For this review, take the finished solid that the model builds, in its own axes (mm). A direction names the side the tool comes from. Round coordinates to 2 decimals unless told otherwise and drop trailing zeros. Write each loop counter-clockwise with the first axis right and the second up, starting at its lowest first coordinate (ties: lowest second). Pieces come first, ordered by that corner, then holes. Notation, with made-up numbers: M 7.5,-2 L 14.5,-2 A3 ccw 14.5,2 Z; hole C 70.25,7 d11. An arc over 180 degrees is marked long. Answer in a Markdown table with one row per item.
Autodesk Inventor part; units mm, degrees
ref_plane "YZ Plane" through (0, 0, 0) normal (1, 0, 0) x (0, 1, 0)
ref_plane "XZ Plane" through (0, 0, 0) normal (0, 1, 0) x (-1, 0, 0)
ref_plane "XY Plane" through (0, 0, 0) normal (0, 0, 1) x (1, 0, 0)
sketch "Sketch2" plane through (0, 0, 0) normal (0, 1, 0) x (-1, 0, 0)
  circle A0 centre (0, 0) radius 10
  dimension "d0" = 20
extrude "Extrusion1" add sketch "Sketch2" along normal blind 20
sketch "Sketch3" plane through (0, 0, 0) normal (0, -1, 0) x (1, 0, 0)
  circle A0 centre (0, 0) radius 4.15
  dimension "d3" = 8.3
extrude "Extrusion2" cut sketch "Sketch3" against normal blind 12.4
sketch "Sketch4" plane through (0, 12.4, 0) normal (0, -1, 0) x (1, 0, 0)
  circle A0 centre (0, 0) radius 4.15
  circle A1 centre (0, 0) radius 3.2
  line L0 (3.2, 0) -> (-1.7, 0)
  line L1 (-1.7, 0) -> (-1.7, -3.7858)
  line L2 (-1.7, 0) -> (-1.7, 3.7858)
  point P0 (-1.7, 2.7111)
  point P1 (-1.7, -2.7111)
  dimension "d16" = 6.4
  dimension "d17" = 4.9
extrude "Extrusion3" cut sketch "Sketch4" against normal blind 6.7 contours A1 L0 L2 | L1 L0 A1
sketch "Sketch8" plane through (0, 0, 0) normal (0, -1, 0) x (1, 0, 0)
  circle A0 centre (0, 0) radius 9.1
  dimension "d18" = 18.2
extrude "Extrusion7" cut sketch "Sketch8" against normal blind 4.5
sketch "Sketch9" plane through (0, 0, 0) normal (0, -1, 0) x (1, 0, 0)
  circle A0 centre (0, 0) radius 10
extrude "Extrusion8" cut sketch "Sketch9" against normal blind 2.8
sketch "Sketch10" plane through (0, 12.4, 0) normal (0, -1, 0) x (1, 0, 0)
  arc A0 (-1.7, -2.7111) -> (-1.7, 2.7111) centre (0, 0) ccw
  line L0 (-1.7, -2.7111) -> (-1.7, 2.7111)
  circle A1 centre (0, 0) radius 4.15
extrude "Extrusion9" cut sketch "Sketch10" against normal blind 0.4
properties part number "RotaryEncoderKnob"
Q1. Take a section at D-D (z = -7.75). State the section outline as (x, y) points, then the cut area to 3 significant figures.
Found:
| item | result |
|---|---|
| outline | M -6.32,2.8 L -4.77,2.8 L -4.77,4.5 L 4.77,4.5 L 4.77,2.8 L 6.32,2.8 L 6.32,20 L -6.32,20 Z |
| area | 201 mm² |
Q2. Take a section at A-A (y = 6.5). State the section outline as (x, z) points.
Found:
| item | result |
|---|---|
| outline | C 0,0 d20; hole C 0,0 d8.3 |
Q3. Take a section at B-B (z = 0). State the section outline as (x, y) points, then the cut area to 3 significant figures.
Found:
| item | result |
|---|---|
| outline | M -10,2.8 L -9.1,2.8 L -9.1,4.5 L -4.15,4.5 L -4.15,12.8 L -1.7,12.8 L -1.7,19.1 L 3.2,19.1 L 3.2,12.8 L 4.15,12.8 L 4.15,4.5 L 9.1,4.5 L 9.1,2.8 L 10,2.8 L 10,20 L -10,20 Z |
| area | 213 mm² |
Q4. Mouldability with a two-part tool opening along X and no side actions: class faces 3 (the face through (2.17, 11.28, 9.76)), 4 (the face through (-4.5, 2.8, -8.1)), 5 (the face through (-1.973, 3.638, -8.884)) as +X half, -X half, draft (parallel to the pull), parting line (faces both ways), or undercut.
Found:
| item | result |
|---|---|
| face 3 | parting line |
| face 4 | draft |
| face 5 | undercut |
Q5. For probe 1 along Z at (x, y) = (0, 8.75); probe 2 along X at (y, z) = (10.75, 0.25); probe 3 along Z at (x, y) = (0, 3.35), list the stretches that pass through material, from the lowest coordinate up.
Found:
| item | result |
|---|---|
| probe 1 | -10 to -4.15, 4.15 to 10 |
| probe 2 | -10 to -4.14, 4.14 to 10 |
| probe 3 | -10 to -9.1, 9.1 to 10 |
Q6. Machinability: for faces 1 (the face through (0, 20, 0)), 2 (the face through (2, 4.5, -4)), which of the approach directions +Z, -Z, +X, -X, +Y, -Y give a long, thin tool a straight path to every point of the face, cutting with its end or side? Answer none if there is none.
Found:
| item | result |
|---|---|
| face 1 | +Z, -Z, +X, -X, +Y |
| face 2 | -Y |
Q7. Take a section at C-C (x = 0). State the section outline as (y, z) points.
Found:
| item | result |
|---|---|
| outline | M 2.8,-10 L 20,-10 L 20,10 L 2.8,10 L 2.8,9.1 L 4.5,9.1 L 4.5,4.15 L 12.8,4.15 L 12.8,3.2 L 19.1,3.2 L 19.1,-3.2 L 12.8,-3.2 L 12.8,-4.15 L 4.5,-4.15 L 4.5,-9.1 L 2.8,-9.1 Z |
Q8. Insertion check: P1, Ø4, axis at x = 0, z = 0, coming from the -Y side; P2, Ø9.5, axis at x = 0, z = 0, coming from the -Y side; P3, Ø3, axis at x = -4.5, y = 11, coming from the +Z side. Each pin has a flat end and moves straight along its axis. Give the tip position at first contact, or say it passes through.
Found:
| item | result |
|---|---|
| P1 | y = 12.8 |
| P2 | y = 4.5 |
| P3 | z = 9.54 |
